Design review of the part built by this model. Coordinates are the model's own, in mm. Face numbers are marked on the shaded views. A direction names the side the tool comes from. Round coordinates to 2 decimals unless told otherwise and drop trailing zeros. Loops run counter-clockwise (first coordinate to the right, second up) from the corner with the lowest first, then second, coordinate; pieces in that order, holes last. Notation, with made-up numbers: (81.25, -22.5) -> (109.25, -22.5) arc R15 cw to (109.25, 1.5) -> close; hole circle Ø7 at (85.5, 33). An arc over 180 degrees is marked (long way). Write each question's results on one line, items separated by ' | '. Start each with the question number.
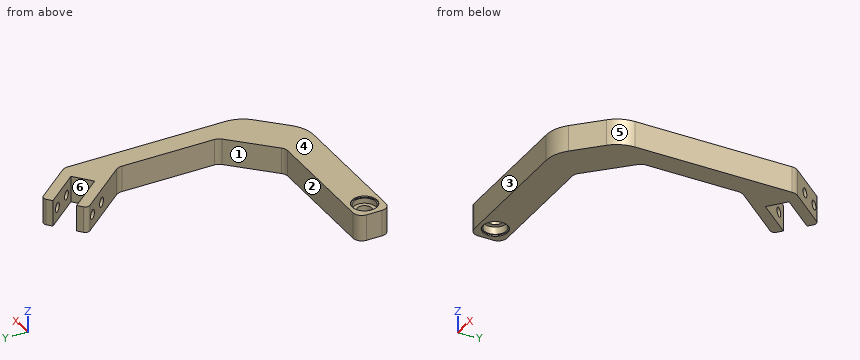
from build123d import *

# Parameters (mm, degrees)
EXTRUDE_1_DEPTH     = 6
CUT_EXTRUDE_1_DEPTH = 122.974454449
SKETCH_3_R          = 3.25
CUT_EXTRUDE_2_DEPTH = 122.974454449
SKETCH_4_R          = 2.1
CUT_EXTRUDE_3_DEPTH = 141.351978867
CHAMFER_1_SIZE      = 20
CHAMFER_2_SIZE      = 20
FILLET_1_R          = 4
FILLET_2_R          = 2
FILLET_3_R          = 15
SKETCH_5_R          = 5.1
CUT_EXTRUDE_4_DEPTH = 3
SKETCH_7_R          = 5.7
CUT_EXTRUDE_6_DEPTH = 0.6
CUT_EXTRUDE_START   = -3
SKETCH_8_R          = 5.1
CUT_EXTRUDE_7_DEPTH = 3
CUT_EXTRUDE_START_2 = -0.6
SKETCH_9_R          = 5.7
CUT_EXTRUDE_8_DEPTH = 0.6
CUT_EXTRUDE_START_3 = -4
SKETCH_6_R          = 5.1
CUT_EXTRUDE_5_DEPTH = 4
FILLET_4_R          = 5


with BuildPart() as part:
    # 草图1 → 凸台-拉伸1 (new, symmetric)
    with BuildSketch(Plane.XY):
        Polygon((0, 0), (15.320888862, 12.855752194), (31.390579105, -6.295358884), (31.390579105, -106.295358884), (-58.609420895, -106.295358884), (-58.609420895, -91.295358884), (21.390579105, -91.295358884), (21.390579105, -25.492299496), align=None)
    extrude(amount=EXTRUDE_1_DEPTH, both=True)

    # 草图2 → 切除-拉伸1 (cut, through all)
    with BuildSketch(Plane.XY.offset(6)):
        Polygon((3.753617771, 3.149659287), (16.609369965, -12.171229575), (24.423023285, -5.614795956), (11.567271091, 9.706092906), align=None)
    extrude(amount=-CUT_EXTRUDE_1_DEPTH, mode=Mode.SUBTRACT)

    # 草图3 → 切除-拉伸2 (cut, through all)
    with BuildSketch(Plane.XY.offset(6)):
        with Locations((-50.609420895, -98.795358884)):
            Circle(SKETCH_3_R)
    extrude(amount=-CUT_EXTRUDE_2_DEPTH, mode=Mode.SUBTRACT)

    # 草图4 → 切除-拉伸3 (cut, through all)
    with BuildSketch(Plane(origin=(15.320888862, 12.855752194, 0), x_dir=(0, 0, -1), z_dir=(0.766044443118977, 0.6427876096865407, 0))):
        with Locations(Location((0, -5, 0), (0, 0, 90))):
            Circle(SKETCH_4_R)
        with Locations(Location((0, -15, 0), (0, 0, 90))):
            Circle(SKETCH_4_R)
    extrude(amount=-CUT_EXTRUDE_3_DEPTH, mode=Mode.SUBTRACT)

    # 倒角1
    chamfer_1_edges = [part.edges().sort_by_distance(p)[0] for p in [
        (21.390579105, -91.295358884, 0),
    ]]
    chamfer(chamfer_1_edges, length=CHAMFER_1_SIZE)

    # 倒角2
    chamfer_2_edges = [part.edges().sort_by_distance(p)[0] for p in [
        (31.390579105, -106.295358884, 0),
    ]]
    chamfer(chamfer_2_edges, length=CHAMFER_2_SIZE)

    # 圆角1
    fillet_1_edges = [part.edges().sort_by_distance(p)[0] for p in [
        (-58.609420895, -106.295358884, 0),
        (-58.609420895, -91.295358884, 0),
        (1.390579105, -91.295358884, 0),
        (21.390579105, -71.295358884, 0),
    ]]
    fillet(fillet_1_edges, radius=FILLET_1_R)

    # 圆角2
    fillet_2_edges = [part.edges().sort_by_distance(p)[0] for p in [
        (0, 0, 0),
        (15.320888862, 12.855752194, 0),
    ]]
    fillet(fillet_2_edges, radius=FILLET_2_R)

    # 圆角3
    fillet_3_edges = [part.edges().sort_by_distance(p)[0] for p in [
        (31.390579105, -86.295358884, 0),
        (11.390579105, -106.295358884, 0),
    ]]
    fillet(fillet_3_edges, radius=FILLET_3_R)

    # 草图5 → 切除-拉伸4 (cut)
    with BuildSketch(Plane.XY.offset(6)):
        with Locations((-50.609420895, -98.795358884)):
            Circle(SKETCH_5_R)
    extrude(amount=-CUT_EXTRUDE_4_DEPTH, mode=Mode.SUBTRACT)

    # 草图7 → 切除-拉伸6 (cut)
    with BuildSketch(Plane.XY.offset(6)):
        with Locations((-50.609420895, -98.795358884)):
            Circle(SKETCH_7_R)
    extrude(amount=-CUT_EXTRUDE_6_DEPTH, mode=Mode.SUBTRACT)

    # 草图8 → 切除-拉伸7 (cut)
    with BuildSketch(Plane(origin=(0, 0, -6), x_dir=(-1, 0, 0), z_dir=(0, 0, -1)).offset(CUT_EXTRUDE_START)):
        with Locations(Location((50.609420895, -98.795358884, 0), (0, 0, 180))):
            Circle(SKETCH_8_R)
    extrude(amount=CUT_EXTRUDE_7_DEPTH, mode=Mode.SUBTRACT)

    # 草图9 → 切除-拉伸8 (cut)
    with BuildSketch(Plane(origin=(0, 0, -6), x_dir=(-1, 0, 0), z_dir=(0, 0, -1)).offset(CUT_EXTRUDE_START_2)):
        with Locations(Location((50.609420895, -98.795358884, 0), (0, 0, 180))):
            Circle(SKETCH_9_R)
    extrude(amount=CUT_EXTRUDE_8_DEPTH, mode=Mode.SUBTRACT)

    # 草图6 → 切除-拉伸5 (cut)
    with BuildSketch(Plane(origin=(0, 0, -6), x_dir=(-1, 0, 0), z_dir=(0, 0, -1)).offset(CUT_EXTRUDE_START_3)):
        with Locations((50.609420895, -98.795358884)):
            Circle(SKETCH_6_R)
    extrude(amount=CUT_EXTRUDE_5_DEPTH, mode=Mode.SUBTRACT)

    # 圆角4
    fillet_4_edges = [part.edges().sort_by_distance(p)[0] for p in [
        (31.390579105, -6.295358884, 0),
        (21.390579105, -25.492299496, 0),
    ]]
    fillet(fillet_4_edges, radius=FILLET_4_R)


solid = part.part
1) Insertion check: pin 1 (1.5 mm diameter, centred on y = -80.5, z = 3, fed in from -X); pin 2 (8 mm diameter, centred on x = -50, y = -98, fed in from +Z); pin 3 (6 mm diameter, centred on x = -50.61, y = -98.8, fed in from -Z) (3 decimals); pin 4 (4 mm diameter, centred on x = 12, z = 3, fed in from +Y) (3 decimals). Each pin has a flat end and moves straight along its axis. Give the tip position at first contact, or say it passes through.
2) To check wall thickness, follow line 1 (Y direction, x = -4, z = 2.25); line 2 (X direction, y = -2, z = 5.75); line 3 (X direction, y = -66.5, z = 1.5). State the ranges of each line that lie inside material, in increasing order. Write a range as from..to.
3) The part is to be moulded in two halves that separate along Y. For the marked faces 4, 5 and 6, say which applies: +Y half, -Y half, draft (parallel to the pull), parting line (faces both ways), or undercut.
4) Take a section at C-C (x = -4.5). Write out the cut boundary in (y, z), plus the area to 3 significant figures.
5) Take a section at A-A (y = -29.5). Write out the cut boundary in (x, z), plus the area to 3 significant figures.
6) For the marked faces 1, 2 and 3, list the 3-axis set-ups (+Z, -Z, +X, -X, +Y, -Y) from which the entire face can be reached by the end or side of a thin tool; tool diameter is ignored.
Geometry check:
1) pin 1: stops at x = 11.44 | pin 2: stops at z = 3 | pin 3: passes through | pin 4: stops at y = 11.725
2) line 1: y = -106.3..-91.3 | line 2: x = 1.68..8.07, 21.39..27.79 | line 3: x = 21.39..31.39
3) face 4: draft | face 5: -Y half | face 6: undercut
4) outline: (-106.3, -6) -> (-91.3, -6) -> (-91.3, 6) -> (-106.3, 6) -> close | area: 180 mm^2
5) outline: (21.39, -6) -> (31.39, -6) -> (31.39, 6) -> (21.39, 6) -> close | area: 120 mm^2
6) face 1: +Z, -Z, -X | face 2: +Z, -Z, -X, +Y | face 3: +Z, -Z, +X, -X, -Y
